Geometry: final body of the model. Coordinates: model frame, mm. Round coordinates to 2 decimals unless told otherwise and drop trailing zeros. Write each loop counter-clockwise with the first axis right and the second up, starting at its lowest first coordinate (ties: lowest second). Pieces come first, ordered by that corner, then holes. Notation, with made-up numbers: (26, -13.75) - (41, -13.75) arc R20 cw to (41, 1.25) - close; hole circle Ø7 at (28, -37). An arc over 180 degrees is marked (long way). Use a Markdown table: item, result. Add a question column.
```python
from build123d import *

# Parameters (mm, degrees)
EXTRUDE_1_DEPTH     = 25
SKETCH_2_R          = 1.5
CUT_EXTRUDE_1_DEPTH = 26.26424494


with BuildPart() as part:
    # 草图1 → 凸台-拉伸1 (new body)
    with BuildSketch(Plane(origin=(0, 0, 0), x_dir=(1, 0, 0), z_dir=(0, 1, 0))):
        Polygon((2.440476282, 1.186342637), (0.19283528, 2.706685776), (-2.247641002, 1.520343139), (-2.440476282, -1.186342637), (-0.19283528, -2.706685776), (2.247641002, -1.520343139), align=None)
    extrude(amount=EXTRUDE_1_DEPTH)

    # 草图2 → 切除-拉伸1 (cut, through all)
    with BuildSketch(Plane.XZ):
        with Locations(Location((0, 0, 0), (0, 0, 270))):
            Circle(SKETCH_2_R)
    extrude(amount=-CUT_EXTRUDE_1_DEPTH, mode=Mode.SUBTRACT)


solid = part.part
```
1) Section B-B, the plane z = -0.25. Return the cut outline in (x, y).
2) Material intervals for L1, parallel to Z at x = 0.9, y = 18; L2, parallel to X at y = 18, z = 0; L3, parallel to X at y = 19.75, z = 0.3, sorted ascending. Write a range as from..to.
3) Section A-A, the plane y = 10.25. Return the cut outline in (x, z).
4) Section D-D, the plane z = -2.3. Return the cut outline in (x, y), then the cut area to 3 significant figures.
5) Section C-C, the plane x = -1.8. Return the cut outline in (y, z).
6) Draft query along Z for faces 1 (the cylindrical face through (0.45, 12.32, -1.43)), 2 (the flat face through (-1.332, 12.325, 1.936)), 3 (the flat face through (2, 0, 0)), 4 (the flat face through (1.332, 12.325, -1.936)). Return one class per face: released by +Z, released by -Z, zero draft, split by the parting line, or undercut.
Output values:
| question | item | result |
|---|---|---|
| 1 | outline | (-2.34, 0) - (-1.48, 0) - (-1.48, 25) - (-2.34, 25) - close; (1.48, 0) - (2.37, 0) - (2.37, 25) - (1.48, 25) - close |
| 2 | L1 | z = -2.23..-1.2, 1.2..2.18 |
| 2 | L2 | x = -2.36..-1.5, 1.5..2.36 |
| 2 | L3 | x = -2.38..-1.47, 1.47..2.33 |
| 3 | outline | (-2.44, 1.19) - (-2.25, -1.52) - (0.19, -2.71) - (2.44, -1.19) - (2.25, 1.52) - (-0.19, 2.71) - close; hole circle Ø3 at (0, 0) |
| 4 | outline | (-0.64, 0) - (0.79, 0) - (0.79, 25) - (-0.64, 25) - close |
| 4 | area | 35.9 mm^2 |
| 5 | outline | (0, -1.74) - (25, -1.74) - (25, 1.62) - (0, 1.62) - close |
| 6 | face 1 | undercut |
| 6 | face 2 | released by +Z |
| 6 | face 3 | zero draft |
| 6 | face 4 | released by -Z |
